from build123d import *

# Parameters (mm, degrees)
SKETCH1_W           = 20
SKETCH1_H           = 100
BOSS_EXTRUDE4_DEPTH = 6
SKETCH1_8_W         = 79
SKETCH1_8_H         = 30
BOSS_EXTRUDE5_DEPTH = 6
SKETCH3_W           = 79
SKETCH3_H           = 10
BOSS_EXTRUDE6_DEPTH = 6
SKETCH6_W           = 20
SKETCH6_H           = 70
BOSS_EXTRUDE8_DEPTH = 6


with BuildPart() as part:
    # Sketch1 → Boss-Extrude4 (new body)
    with BuildSketch(Plane.XY):
        with Locations((10, 50)):
            Rectangle(SKETCH1_W, SKETCH1_H)
    extrude(amount=BOSS_EXTRUDE4_DEPTH)

    # Sketch1_8 → Boss-Extrude5 (add)
    with BuildSketch(Plane.XY):
        with Locations((39.5, -15)):
            Rectangle(SKETCH1_8_W, SKETCH1_8_H)
    extrude(amount=BOSS_EXTRUDE5_DEPTH)

    # Sketch3 → Boss-Extrude6 (add)
    with BuildSketch(Plane.XY.offset(6)):
        with Locations((39.5, -15)):
            Rectangle(SKETCH3_W, SKETCH3_H)
    extrude(amount=BOSS_EXTRUDE6_DEPTH)

    # Sketch6 → Boss-Extrude8 (add)
    with BuildSketch(Plane.XY.offset(6)):
        with Locations((10, 65)):
            Rectangle(SKETCH6_W, SKETCH6_H)
    extrude(amount=BOSS_EXTRUDE8_DEPTH)


solid = part.part
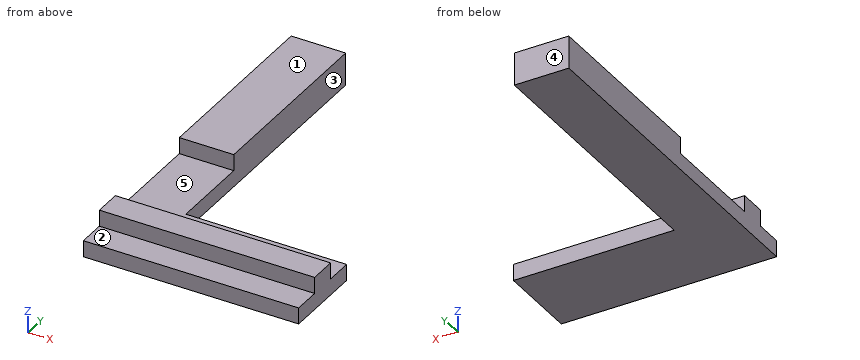
Geometry: final body of the model. Coordinates: model frame, mm. Face numbers are marked on the shaded views. A direction names the side the tool comes from. Give positions to 0.01 mm unless a question says otherwise; leave off trailing zeros. Write each loop counter-clockwise with the first axis right and the second up, starting at its lowest first coordinate (ties: lowest second). Pieces come first, ordered by that corner, then holes.
(1) Ray query, line 1 (Y direction, x = 31, z = 7.25); line 2 (X direction, y = 51.5, z = 3.75); line 3 (Z direction, x = 16.5, y = 15.5). Return the intervals inside material, ascending.
(2) Cut plane A-A, the plane z = 8.5. Return loops of the section in (x, y).
(3) First-contact query: P1, Ø1, axis at y = 62, z = 9, coming from the -X side; P2, Ø1.8, axis at x = 43.5, z = 2, coming from the +Y side; P3, Ø3.5, axis at y = 39.5, z = 5, coming from the +X side; P4, Ø3, axis at x = 23, z = 10, coming from the -Y side. Flat tips, straight axial feed; report the tip coordinate or a pass-through.
(4) Mould query, pull axis Y, two halves, no side actions, for the marked faces 3, 4 and 5. Classes: released by +Y, released by -Y, zero draft, split by the parting line, or undercut.
(5) Access query for the marked faces 1 and 2. Directions: +Z, -Z, +X, -X, +Y, -Y. A direction counts if a zero-diameter tool reaches every point of the face in a straight line with its end or side. Return the directions, or none.
(6) Cut plane B-B, the plane x = 12. Return loops of the section in (y, z), then the cut area to 3 significant figures.
(7) Cut plane C-C, the plane y = 61. Return loops of the section in (x, z), then the cut area to 3 significant figures.
(8) Cut plane D-D, the plane x = 35. Return loops of the section in (y, z).
Values follow:
1. line 1: y = -20 to -10
1. line 2: x = 0 to 20
1. line 3: z = 0 to 6
2. outline: (0, -20) - (79, -20) - (79, -10) - (0, -10) - close; (0, 30) - (20, 30) - (20, 100) - (0, 100) - close
3. P1: stops at x = 0
3. P2: stops at y = 0
3. P3: stops at x = 20
3. P4: stops at y = -20
4. face 3: zero draft
4. face 4: released by +Y
4. face 5: undercut
5. face 1: +Z, +X, -X, +Y, -Y
5. face 2: +Z, +X, -X, -Y
6. outline: (-30, 0) - (100, 0) - (100, 12) - (30, 12) - (30, 6) - (-10, 6) - (-10, 12) - (-20, 12) - (-20, 6) - (-30, 6) - close
6. area: 1,260 mm2
7. outline: (0, 0) - (20, 0) - (20, 12) - (0, 12) - close
7. area: 240 mm2
8. outline: (-30, 0) - (0, 0) - (0, 6) - (-10, 6) - (-10, 12) - (-20, 12) - (-20, 6) - (-30, 6) - close
